```python
from build123d import *

# Parameters (mm, degrees)
BOSS_EXTRUDE1_DEPTH = 146.05


with BuildPart() as part:
    # Sketch1 → Boss-Extrude1 (new body)
    with BuildSketch(Plane(origin=(0, 0, 0), x_dir=(1, 0, 0), z_dir=(0, 1, 0))):
        Polygon((0, 38.1), (-6.35, 0), (-6.35, -5.08), (-3.175, -5.08), (-3.175, 0), (-1.5875, 0), (-1.5875, 9.262228966), (1.5875, 9.262228966), (1.5875, 0), (3.175, 0), (3.175, -5.08), (6.35, -5.08), (6.35, 0), align=None)
    extrude(amount=BOSS_EXTRUDE1_DEPTH)


solid = part.part
```
Model file for the job. Use its own axes, mm. A direction names the side the tool comes from. Coordinates: 2 decimals unless noted, no trailing zeros. Order: outer loops, then holes, each group sorted by start corner. A loop starts at its lowest first (then second) coordinate and runs counter-clockwise, first axis right, second up. Notation, with made-up numbers: M -35,80.5 L -9,80.5 A14 cw -9,103.5 Z; hole C -17,-11 d9. An arc over 180 degrees is marked long. Answer as CSV lines item,"result".
(1) Pull direction Z, two halves, no side cores. Call faces 1 (the flat face through (0, 146.05, -12)), 2 (the flat face through (-3.13, 72, -19.32)), 3 (the flat face through (-5, 72, 5.08)): +Z half, -Z half, draft (parallel to the pull), parting line (faces both ways), or undercut.
Geometry says:
face 1,"draft"
face 2,"-Z half"
face 3,"+Z half"
(2) 3-axis set-ups, long thin cutter, end or side, ignore diameter. For faces 4 (the flat face through (0, 72, -9.262)), 5 (the flat face through (3.22, 72, -18.78)): which of +Z, -Z, +X, -X, +Y, -Y reach the whole face in a straight line?
Geometry says:
face 4,"+Z, +Y, -Y"
face 5,"-Z, +X, +Y, -Y"
(3) Band-saw the part on D-D, the plane z = -28. List the corners of the cut face in (x, y).
Geometry says:
outline,"M -1.68,0 L 1.68,0 L 1.68,146.05 L -1.68,146.05 Z"
(4) Flat gauge pins, fed straight in: pin 1 (1.7 mm diameter, centred on x = -2, y = 105, fed in from +Z); pin 2 (10 mm diameter, centred on y = 33, z = -15.5, fed in from +X); pin 3 (4 mm diameter, centred on y = 127.5, z = -30.5, fed in from -X). Where does each tip first touch, or does it go through?
Geometry says:
pin 1,"stops at z = 0"
pin 2,"stops at x = 4.6"
pin 3,"stops at x = -1.6"
(5) Band-saw the part on C-C, the plane z = -17. List the corners of the cut face in (x, y), then the cut area to 3 significant figures.
Geometry says:
outline,"M -3.52,0 L 3.52,0 L 3.52,146.05 L -3.52,146.05 Z"
area,"1,030 mm2"
(6) Band-saw the part on B-B, the plane z = -2.5. List the corners of the cut face in (x, y).
Geometry says:
outline,"M -5.93,0 L -1.59,0 L -1.59,146.05 L -5.93,146.05 Z; M 1.59,0 L 5.93,0 L 5.93,146.05 L 1.59,146.05 Z"
(7) Wall check: line 1 along X through (y, z) = (61.5, 1) (3 decimals); line 2 along X through (y, z) = (21.5, -1.5); line 3 along X through (y, z) = (28, -28). Give the ranges that are in metal, low to high.
Geometry says:
line 1,"x = -6.35 to -3.175, 3.175 to 6.35"
line 2,"x = -6.1 to -1.59, 1.59 to 6.1"
line 3,"x = -1.68 to 1.68"
